```python
from build123d import *

# Parameters (mm, degrees)
SKETCH1_W           = 70
SKETCH1_H           = 20
BOSS_EXTRUDE1_DEPTH = 5
FILLET1_R           = 10
SKETCH2_R           = 2.15
CUT_EXTRUDE1_DEPTH  = 10
BOSS_EXTRUDE2_DEPTH = 20
SKETCH6_R           = 6
CUT_EXTRUDE3_DEPTH  = 20


with BuildPart() as part:
    # Sketch1 → Boss-Extrude1 (new body)
    with BuildSketch(Plane(origin=(0, 0, 0), x_dir=(1, 0, 0), z_dir=(0, 1, 0))):
        with Locations((-22.239915074, 10)):
            Rectangle(SKETCH1_W, SKETCH1_H)
    extrude(amount=BOSS_EXTRUDE1_DEPTH)

    # Fillet1
    fillet1_edges = [part.edges().sort_by_distance(p)[0] for p in [
        (12.760084926, 2.5, 0),
        (12.760084926, 2.5, -20),
        (-57.239915074, 2.5, 0),
        (-57.239915074, 2.5, -20),
    ]]
    fillet(fillet1_edges, radius=FILLET1_R - 0.0001)  # a hair under: the kernel refuses the full size

    # Sketch2 → Cut-Extrude1 (cut)
    with BuildSketch(Plane(origin=(0, 5, 0), x_dir=(1, 0, 0), z_dir=(0, 1, 0))):
        with Locations(Location((-47.239915074, 10, 0), (0, 0, 270))):
            Circle(SKETCH2_R)
        with Locations(Location((2.760084926, 10, 0), (0, 0, 270))):
            Circle(SKETCH2_R)
    extrude(amount=-CUT_EXTRUDE1_DEPTH, mode=Mode.SUBTRACT)

    # Sketch3 → Boss-Extrude2 (add)
    with BuildSketch(Plane(origin=(0, 0, -20), x_dir=(-1, 0, 0), z_dir=(0, 0, -1))):
        with BuildLine():
            Line((14.239915074, 5), (30.239915074, 5))
            ThreePointArc((30.239915074, 5), (22.239915074, 13), (14.239915074, 5))
        make_face()
    extrude(amount=-BOSS_EXTRUDE2_DEPTH)

    # Sketch6 → Cut-Extrude3 (cut)
    with BuildSketch(Plane(origin=(0, 0, -20), x_dir=(-1, 0, 0), z_dir=(0, 0, -1))):
        with Locations((22.239915074, 5)):
            Circle(SKETCH6_R)
    extrude(amount=-CUT_EXTRUDE3_DEPTH, mode=Mode.SUBTRACT)


solid = part.part
```
Can you work these out from the model? Positions are in its coordinate system, mm. A direction names the side the tool comes from. Coordinates: 2 decimals unless noted, no trailing zeros. Loops run counter-clockwise (first coordinate to the right, second up) from the corner with the lowest first, then second, coordinate; pieces in that order, holes last.
1) For pin 1 (5 mm diameter, centred on x = -47.24, z = -10, fed in from +Y); pin 2 (2 mm diameter, centred on x = -16, z = -3.5, fed in from +Y); pin 3 (1.5 mm diameter, centred on y = 6, z = -16.5, fed in from -X), each with a flat end and sliding along its axis, tell me the tip position at first contact or that it passes through.
2) Imagine slicing it at B-B on z = -9. List the corners of the cut face in (x, y) for me, plus the area to 3 significant figures.
3) Imagine slicing it at D-D on x = -43. List the corners of the cut face in (y, z) for me, plus the area to 3 significant figures.
4) I need wall thicknesses on probe 1 along X at (y, z) = (2.35, -10); probe 2 along X at (y, z) = (1.4, -10); probe 3 along X at (y, z) = (10, -5). Which ranges of each line are inside material? Lowest first, please.
5) Imagine slicing it at C-C on z = -4.25. List the corners of the cut face in (x, y) for me.
6) Imagine slicing it at A-A on y = 6.25. List the corners of the cut face in (x, z) for me, plus the area to 3 significant figures.
7) Thinking about a two-plate mould opening in X: for faces 1 (the flat face through (-28, 2, -20)), 2 (the cylindrical face through (9.9, 2.5, -17)), 3 (the cylindrical face through (3.41, 2.54, -7.95)), 4 (the cylindrical face through (-22.4, 13, -10.1)), which applies, pulls with the +X half, pulls with the -X half, needs draft (parallel to the pull), parting line crosses it, or undercut?
8) Which directions (+Z, -Z, +X, -X, +Y, -Y) give clear straight access to the entire face, cutting with the end or side of a thin tool? Please do faces 5 (the flat face through (-42, 0, -10)), 6 (the flat face through (-1, 5, -10)), 7 (the flat face through (-44, 5, -10)).
Completed:
1. pin 1: stops at y = 5
1. pin 2: stops at y = 11.05
1. pin 3: stops at x = -30.24
2. outline: (-57.19, 0) - (-49.14, 0) - (-49.14, 5) - (-57.19, 5) - close; (-45.34, 0) - (-25.56, 0) arc R6 cw (long way) to (-18.92, 0) - (0.86, 0) - (0.86, 5) - (-14.24, 5) arc R8 ccw to (-30.24, 5) - (-45.34, 5) - close; (4.66, 0) - (12.71, 0) - (12.71, 5) - (4.66, 5) - close
2. area: 303 mm2
3. outline: (0, -20) - (5, -20) - (5, 0) - (0, 0) - close
3. area: 100 mm2
4. probe 1: x = -57.24 to -49.39, -45.09 to -27.62, -16.86 to 0.61, 4.91 to 12.76
4. probe 2: x = -57.24 to -49.39, -45.09 to -27.04, -17.44 to 0.61, 4.91 to 12.76
4. probe 3: x = -28.48 to -25.56, -18.92 to -15.99
5. outline: (-55.42, 0) - (-25.56, 0) arc R6 cw (long way) to (-18.92, 0) - (10.94, 0) - (10.94, 5) - (-14.24, 5) arc R8 ccw to (-30.24, 5) - (-55.42, 5) - close
6. outline: (-30.14, -20) - (-28.11, -20) - (-28.11, 0) - (-30.14, 0) - close; (-16.37, -20) - (-14.34, -20) - (-14.34, 0) - (-16.37, 0) - close
6. area: 81.3 mm2
7. face 1: needs draft
7. face 2: pulls with the +X half
7. face 3: undercut
7. face 4: parting line crosses it
8. face 5: +Z, -Z, +X, -X, -Y
8. face 6: +Z, -Z, +X, +Y
8. face 7: +Z, -Z, -X, +Y
